Source: CAD feature listing. Evaluate the final solid. Frame: model axes, mm. A direction names the side the tool comes from. Give positions to 0.01 mm unless a question says otherwise; leave off trailing zeros. Loops run counter-clockwise (first coordinate to the right, second up) from the corner with the lowest first, then second, coordinate; pieces in that order, holes last.
Autodesk Inventor part; units mm, degrees
ref_plane "YZ Plane" through (0, 0, 0) normal (1, 0, 0) x (0, 1, 0)
ref_plane "XZ Plane" through (0, 0, 0) normal (0, 1, 0) x (-1, 0, 0)
ref_plane "XY Plane" through (0, 0, 0) normal (0, 0, 1) x (1, 0, 0)
sketch "Sketch1" plane through (0, 0, 0) normal (0, 1, 0) x (-1, 0, 0)
  circle A0 centre (0, 0) radius 15.55
  circle A1 centre (0, 0) radius 14.75
  dimension "d0" = 31.1
  dimension "d1" = 29.5
sketch "Sketch2" plane through (0, 0, 0) normal (0, 0, 1) x (1, 0, 0)
  line L0 (-445, 1700) -> (-150, 1700)
  line L1 (0, 1550) -> (0, 0)
  arc A0 (0, 1550) -> (-150, 1700) centre (-150, 1550) ccw
  point P0 (0, 1700)
  dimension "d4" = 445
  dimension "d6" = 150
  dimension "d9" = 1700
sweep "Sweep1" add profiles "Sketch1" path "Sketch2"
properties part number "SP13V1 Tubo Baranda" material "Acero, carbono"
1) Cut plane B-B (y = 780.5). Return loops of the section in (x, z).
Checks:
outline: circle Ø31.1 at (0, 0); hole circle Ø29.5 at (0, 0)
2) Cut plane C-C (x = -261). Return loops of the section in (y, z), and give its area (3 significant figures).
Checks:
outline: circle Ø31.1 at (1700, 0); hole circle Ø29.5 at (1700, 0)
area: 76.2 mm2
3) Reachability of faces 1 (the flat face through (12, 0, 9)), 2 (the cylindrical face through (-295.44, 1685.93, -4.43)) from +Z, -Z, +X, -X, +Y, -Y: full face, straight path, thin tool, end or side. Return the list, or none.
Checks:
face 1: +Z, -Z, +X, -X, -Y
face 2: -X
4) Contact query for flat-ended pins moving along their axis: P1, Ø10, axis at x = -133, z = -8.5, coming from the -Y side; P2, Ø5, axis at y = 1500.5, z = -1.5, coming from the -X side; P3, Ø2, axis at y = 698, z = 9.5, coming from the -X side. Output: stop coordinate, or through.
Checks:
P1: stops at y = 1683.6
P2: stops at x = -15.55
P3: stops at x = -13.02
5) Ray query, probe 1 along X at (y, z) = (392, 2); probe 2 along Z at (x, y) = (0, 538); probe 3 along X at (y, z) = (451.5, -0.5). Return the intervals inside material, ascending.
Checks:
probe 1: x = -15.42 to -14.61, 14.61 to 15.42
probe 2: z = -15.55 to -14.75, 14.75 to 15.55
probe 3: x = -15.54 to -14.74, 14.74 to 15.54
6) Cut plane A-A (z = 0). Return loops of the section in (x, y), and give its area (3 significant figures).
Checks:
outline: (-445, 1684.45) - (-150, 1684.45) arc R134.45 cw to (-15.55, 1550) - (-15.55, 0) - (-14.75, 0) - (-14.75, 1550) arc R135.25 ccw to (-150, 1685.25) - (-445, 1685.25) - close; (-445, 1714.75) - (-150, 1714.75) arc R164.75 cw to (14.75, 1550) - (14.75, 0) - (15.55, 0) - (15.55, 1550) arc R165.55 ccw to (-150, 1715.55) - (-445, 1715.55) - close
area: 3,330 mm2
7) Pull-direction query (X, two-part tool) for faces 3 (the cylindrical face through (-14.07, 764.15, -4.43)), 4 (the cylindrical face through (-295.435, 1685.168, -4.671)), 5 (the flat face through (-445, 1688, -9)), 6 (the cylindrical face through (3.37, 764.15, 15.18)); classes: released by +X, released by -X, zero draft, split by the parting line, or undercut.
Checks:
face 3: undercut
face 4: zero draft
face 5: released by -X
face 6: split by the parting line
